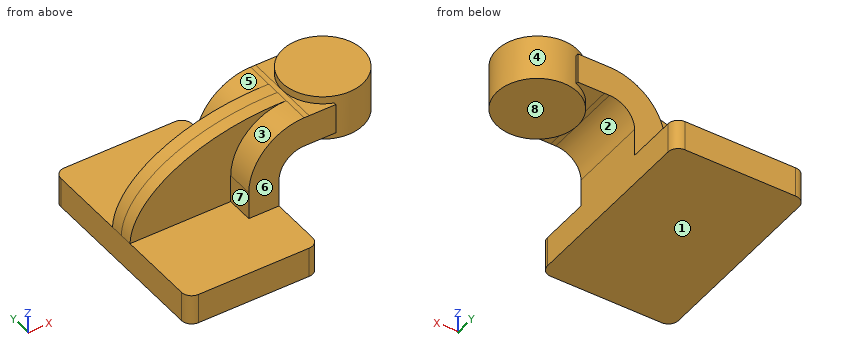
from build123d import *

# Parameters (mm, degrees)
F1_DEPTH = 63.5
F0_W     = 16.733868
F0_H     = 19.049999
F2_DEPTH = 25.4
F3_DEPTH = 8.2804
F0_W_2   = 25.4
F0_H_2   = 28.575
F5_R     = 6.35


with BuildPart() as f1:
    # F0 (on Front) → F1 (new body, symmetric)
    with BuildSketch(Plane.XZ):
        Polygon((41.275, -9.525), (41.275, 9.525), (22.225001, 9.525), (-41.275, 9.525), (-41.275, -9.525), align=None)
    extrude(amount=F1_DEPTH, both=True)

    # F0 (on Front) → F2 (join, symmetric)
    with BuildSketch(Plane.XZ):
        with BuildLine():
            Line((22.225001, 9.525), (41.275, 9.525))
            Line((41.275, 9.525), (41.275, 27.0002))
            ThreePointArc((41.275, 27.0002), (45.92468, 38.22552), (57.15, 42.8752))
            Line((57.15, 42.8752), (60.325, 42.8752))
            Line((60.325, 42.8752), (60.325, 61.925199))
            Line((60.325, 61.925199), (57.15, 61.925199))
            ThreePointArc((57.15, 61.925199), (32.454296, 51.695904), (22.225001, 27.0002))
            Line((22.225001, 27.0002), (22.225001, 9.525))
        make_face()
        with Locations((68.691934, 52.400199)):
            Rectangle(F0_W, F0_H)
    extrude(amount=F2_DEPTH, both=True)

    # F0 (on Front) → F3 (join, symmetric)
    with BuildSketch(Plane.XZ):
        with BuildLine():
            Line((-41.275, 9.525), (22.225001, 9.525))
            Line((22.225001, 9.525), (22.225001, 27.0002))
            ThreePointArc((22.225001, 27.0002), (32.454296, 51.695904), (57.15, 61.925199))
            add(Edge.make_bspline(
                [(-41.275, 9.525), (-40.269591, 37.765782), (0, 63.221171), (57.15, 61.925199)],
                knots=[0, 0, 0, 0, 111.504536, 111.504536, 111.504536, 111.504536], degree=3))
        make_face()
    extrude(amount=F3_DEPTH, both=True)

    # F0 (on Front) → F4 (revolve)
    with BuildSketch(Plane.XZ):
        with Locations((98.425, 52.3875)):
            Rectangle(F0_W_2, F0_H_2)
    revolve(axis=Axis((85.725, 0, 52.3875), (0, 0, 1)))

    # F5
    f5_edges = [f1.edges().sort_by_distance(p)[0] for p in [
        (41.275, -63.5, 0),
        (-41.275, -63.5, 0),
        (41.275, 63.5, 0),
        (-41.275, 63.5, 0),
    ]]
    fillet(f5_edges, radius=F5_R)


solid = f1.part
The listing builds one solid part. Answer for the finished solid, in the listing's coordinates (mm). Face numbers are marked on the shaded views. A direction names the side the tool comes from. Round coordinates to 2 decimals unless told otherwise and drop trailing zeros. Order: outer loops, then holes, each group sorted by start corner. A loop starts at its lowest first (then second) coordinate and runs counter-clockwise, first axis right, second up. Notation, with made-up numbers: (89.5, -13) -> (93.5, -13) arc R16 ccw to (93.5, 1) -> close; hole circle Ø3 at (-23, -12.75). An arc over 180 degrees is marked (long way). Write each question's results on one line, items separated by ' | '. Start each with the question number.
Q1. Find section A-A (z = -5). Determine the outline of the cut face in (x, y) (3 decimals), then the cut area to 3 significant figures.
Q2. Find section B-B (y = 27.5). Determine the outline of the cut face in (x, z) (3 decimals).
Q3. Each of these flat-tipped pins is pushed along its axis until it touches: pin 1 (5 mm diameter, centred on y = 15, z = 14.5, fed in from -X) (3 decimals); pin 2 (15.5 mm diameter, centred on x = -15.5, z = 26, fed in from +Y); pin 3 (3.5 mm diameter, centred on x = 58, y = -4, fed in from +Z). Where does it stop, or does it pass through?
Q4. The mould has two halves that part along X. Classify the marked faces 1, 2, 3 and 4: pulls with the +X half, pulls with the -X half, needs draft (parallel to the pull), parting line crosses it, or undercut.
Q5. Straight lines are drawn through the part: probe 1 along Y at (x, z) = (-15, 35); probe 2 along Y at (x, z) = (58.5, 55); probe 3 along X at (y, z) = (7.5, -2) (3 decimals). For each, find the intervals that lie inside material, in ascending order. Write a range as from..to.
Q6. Which of the six approach directions +Z, -Z, +X, -X, +Y, -Y give full straight-line access (tool end or side, diameter ignored) to the marked faces 5, 6, 7 and 8?
Worked answers:
1) outline: (-41.275, -57.15) arc R6.35 ccw to (-34.925, -63.5) -> (34.925, -63.5) arc R6.35 ccw to (41.275, -57.15) -> (41.275, 57.15) arc R6.35 ccw to (34.925, 63.5) -> (-34.925, 63.5) arc R6.35 ccw to (-41.275, 57.15) -> close | area: 10,400 mm2
2) outline: (-41.275, -9.525) -> (41.275, -9.525) -> (41.275, 9.525) -> (-41.275, 9.525) -> close
3) pin 1: stops at x = 22.225 | pin 2: stops at y = 8.28 | pin 3: stops at z = 61.94
4) face 1: needs draft | face 2: undercut | face 3: pulls with the -X half | face 4: undercut
5) probe 1: y = -8.28..8.28 | probe 2: y = -25.4..25.4 | probe 3: x = -41.275..41.275
6) face 5: +Z, -X, +Y | face 6: +Z, +X, -X, -Y | face 7: +Z, -X, -Y | face 8: -Z, +X, +Y, -Y
